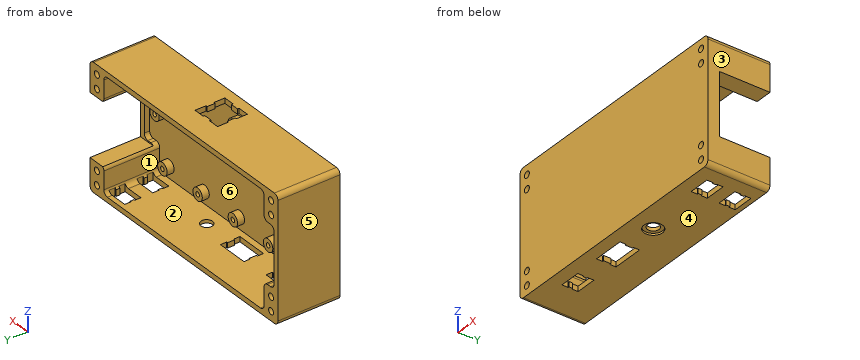
from build123d import *

# Parameters (mm, degrees)
EXTRUDE_1_DEPTH            = 40
CUT_EXTRUDE_1_DEPTH        = 36
EXTRUDE_2_DEPTH            = 36
SKETCH_4_R                 = 2.1
CUT_EXTRUDE_2_DEPTH        = 98.979589711
SKETCH_5_R                 = 4
SKETCH_5_R_2               = 1.5
EXTRUDE_3_DEPTH            = 4.5
PATTERN_LINEAR_1_COUNT     = 3
PATTERN_LINEAR_1_PITCH     = 30
PATTERN_LINEAR_1_COL_COUNT = 3
PATTERN_LINEAR_1_COL_PITCH = 30
SKETCH_6_R                 = 4
SKETCH_6_R_2               = 1.5
EXTRUDE_4_DEPTH            = 4.5
FILLET_1_R                 = 3
SKETCH_7_W                 = 40
SKETCH_7_H                 = 40
CUT_EXTRUDE_3_DEPTH        = 25
CUT_EXTRUDE_4_DEPTH        = 10
SKETCH_9_R                 = 3.75
CUT_EXTRUDE_5_DEPTH        = 3.3
SKETCH_10_R                = 6
CUT_EXTRUDE_6_DEPTH        = 1.2
CUT_EXTRUDE_7_REACH        = 122


with BuildPart() as part:
    # Эскиз1 → Бобышка-Вытянуть1 (new body)
    with BuildSketch(Plane(origin=(0, 0, 0), x_dir=(1, 0, 0), z_dir=(0, 1, 0))):
        with BuildLine():
            Line((-77, -40), (77, -40))
            ThreePointArc((77, -40), (79.121320344, -39.121320344), (80, -37))
            Line((80, -37), (80, 37))
            ThreePointArc((80, 37), (79.121320344, 39.121320344), (77, 40))
            Line((77, 40), (-77, 40))
            ThreePointArc((-77, 40), (-79.121320344, 39.121320344), (-80, 37))
            Line((-80, 37), (-80, -37))
            ThreePointArc((-80, -37), (-79.121320344, -39.121320344), (-77, -40))
        make_face()
    extrude(amount=EXTRUDE_1_DEPTH)

    # Эскиз2 → Вырез-Вытянуть1 (cut)
    with BuildSketch(Plane(origin=(0, 40, 0), x_dir=(1, 0, 0), z_dir=(0, 1, 0))):
        with BuildLine():
            Line((-75.75, -36.7), (75.75, -36.7))
            ThreePointArc((75.75, -36.7), (76.457106781, -36.407106781), (76.75, -35.7))
            Line((76.75, -35.7), (76.75, 35.7))
            ThreePointArc((76.75, 35.7), (76.457106781, 36.407106781), (75.75, 36.7))
            Line((75.75, 36.7), (-75.75, 36.7))
            ThreePointArc((-75.75, 36.7), (-76.457106781, 36.407106781), (-76.75, 35.7))
            Line((-76.75, 35.7), (-76.75, -35.7))
            ThreePointArc((-76.75, -35.7), (-76.457106781, -36.407106781), (-75.75, -36.7))
        make_face()
    extrude(amount=-CUT_EXTRUDE_1_DEPTH, mode=Mode.SUBTRACT)

    # Эскиз3 → Бобышка-Вытянуть2 (add)
    with BuildSketch(Plane(origin=(0, 4, 0), x_dir=(1, 0, 0), z_dir=(0, 1, 0))):
        with BuildLine():
            Line((-76.75, -36.7), (-68.2, -36.7))
            Line((-68.2, -36.7), (-68.2, -22.15))
            ThreePointArc((-68.2, -22.15), (-69.078679656, -20.028679656), (-71.2, -19.15))
            Line((-71.2, -19.15), (-76.75, -19.15))
            Line((-76.75, -19.15), (-76.75, -36.7))
        make_face()
        with BuildLine():
            Line((-68.2, 36.7), (-68.2, 22.15))
            ThreePointArc((-68.2, 22.15), (-69.078679656, 20.028679656), (-71.2, 19.15))
            Line((-71.2, 19.15), (-76.75, 19.15))
            Line((-76.75, 19.15), (-76.75, 36.7))
            Line((-76.75, 36.7), (-68.2, 36.7))
        make_face()
        with BuildLine():
            Line((76.75, 36.7), (68.2, 36.7))
            Line((68.2, 36.7), (68.2, 22.15))
            ThreePointArc((68.2, 22.15), (69.078679656, 20.028679656), (71.2, 19.15))
            Line((71.2, 19.15), (76.75, 19.15))
            Line((76.75, 19.15), (76.75, 36.7))
        make_face()
        with BuildLine():
            Line((68.2, -36.7), (68.2, -22.15))
            ThreePointArc((68.2, -22.15), (69.078679656, -20.028679656), (71.2, -19.15))
            Line((71.2, -19.15), (76.75, -19.15))
            Line((76.75, -19.15), (76.75, -36.7))
            Line((76.75, -36.7), (68.2, -36.7))
        make_face()
    extrude(amount=EXTRUDE_2_DEPTH)

    # Эскиз4 → Вырез-Вытянуть2 (cut, through all)
    with BuildSketch(Plane(origin=(0, 40, 0), x_dir=(1, 0, 0), z_dir=(0, 1, 0))):
        with Locations(Location((-74.15, -34, 0), (0, 0, 270))):
            Circle(SKETCH_4_R)
        with Locations(Location((-74.15, 34, 0), (0, 0, 90))):
            Circle(SKETCH_4_R)
        with Locations(Location((74.15, 34, 0), (0, 0, 270))):
            Circle(SKETCH_4_R)
        with Locations(Location((74.15, -34, 0), (0, 0, 90))):
            Circle(SKETCH_4_R)
        with Locations(Location((-74.15, -25.1, 0), (0, 0, 270))):
            Circle(SKETCH_4_R)
        with Locations(Location((-74.15, 25.1, 0), (0, 0, 90))):
            Circle(SKETCH_4_R)
        with Locations(Location((74.15, 25.1, 0), (0, 0, 270))):
            Circle(SKETCH_4_R)
        with Locations(Location((74.15, -25.1, 0), (0, 0, 90))):
            Circle(SKETCH_4_R)
    extrude(amount=-CUT_EXTRUDE_2_DEPTH, mode=Mode.SUBTRACT)

    # Эскиз5 → Бобышка-Вытянуть3 (add)
    # profile 1 of 2: a face of its own
    with BuildSketch(Plane(origin=(0, 4, 0), x_dir=(1, 0, 0), z_dir=(0, 1, 0))):
        with Locations(Location((0, -29, 0), (0, 0, 90))):
            Circle(SKETCH_5_R)
        with Locations(Location((0, -29, 0), (0, 0, 270))):
            Circle(SKETCH_5_R_2, mode=Mode.SUBTRACT)
    # profile 2 of 2: a face of its own
    with BuildSketch(Plane(origin=(0, 4, 0), x_dir=(1, 0, 0), z_dir=(0, 1, 0))):
        with Locations(Location((0, 29, 0), (0, 0, 90))):
            Circle(SKETCH_5_R)
        with Locations(Location((0, 29, 0), (0, 0, 270))):
            Circle(SKETCH_5_R_2, mode=Mode.SUBTRACT)
    extrude_3 = extrude(amount=EXTRUDE_3_DEPTH)

    # Линейный массив1: Бобышка-Вытянуть3 ×3
    with Locations(*[(i * PATTERN_LINEAR_1_PITCH, 0, 0) for i in range(1, PATTERN_LINEAR_1_COUNT)]):
        add(extrude_3)

    # Линейный массив1 col: Бобышка-Вытянуть3 ×3
    with Locations(*[(-i * PATTERN_LINEAR_1_COL_PITCH, 0, 0) for i in range(1, PATTERN_LINEAR_1_COL_COUNT)]):
        add(extrude_3)

    # Эскиз6 → Бобышка-Вытянуть4 (add)
    # profile 1 of 2: a face of its own
    with BuildSketch(Plane(origin=(0, 4, 0), x_dir=(1, 0, 0), z_dir=(0, 1, 0))):
        with Locations(Location((-68, 0, 0), (0, 0, 90))):
            Circle(SKETCH_6_R)
        with Locations(Location((-68, 0, 0), (0, 0, 270))):
            Circle(SKETCH_6_R_2, mode=Mode.SUBTRACT)
    # profile 2 of 2: a face of its own
    with BuildSketch(Plane(origin=(0, 4, 0), x_dir=(1, 0, 0), z_dir=(0, 1, 0))):
        with Locations(Location((68, 0, 0), (0, 0, 90))):
            Circle(SKETCH_6_R)
        with Locations(Location((68, 0, 0), (0, 0, 90))):
            Circle(SKETCH_6_R_2, mode=Mode.SUBTRACT)
    extrude(amount=EXTRUDE_4_DEPTH)

    # Скругление1
    fillet_1_edges = [part.edges().sort_by_distance(p)[0] for p in [
        (68.2, 22, 36.7),
        (76.75, 22, 19.15),
        (-76.75, 22, 19.15),
        (-68.2, 22, 36.7),
        (-68.2, 22, -36.7),
        (-76.75, 22, -19.15),
        (76.75, 22, -19.15),
        (68.2, 22, -36.7),
    ]]
    fillet(fillet_1_edges, radius=FILLET_1_R)

    # Эскиз7 → Вырез-Вытянуть3 (cut)
    with BuildSketch(Plane(origin=(80, 0, 0), x_dir=(0, 0, -1), z_dir=(1, 0, 0))):
        with Locations((0, 27.5)):
            Rectangle(SKETCH_7_W, SKETCH_7_H)
    extrude(amount=-CUT_EXTRUDE_3_DEPTH, mode=Mode.SUBTRACT)

    # Эскиз8 → Вырез-Вытянуть4 (cut)
    with BuildSketch(Plane(origin=(0, 0, -40), x_dir=(-1, 0, 0), z_dir=(0, 0, -1))):
        Polygon((-54.5, 18.9), (-67.9, 18.9), (-67.9, 14.9), (-67.2, 14.9), (-67.2, 12.5), (-67.9, 12.5), (-67.9, 8.5), (-54.5, 8.5), (-54.5, 12.5), (-55.2, 12.5), (-55.2, 14.9), (-54.5, 14.9), align=None)
        Polygon((55.5, 18.9), (42.1, 18.9), (42.1, 14.9), (42.8, 14.9), (42.8, 12.5), (42.1, 12.5), (42.1, 8.5), (55.5, 8.5), (55.5, 12.5), (54.8, 12.5), (54.8, 14.9), (55.5, 14.9), align=None)
        Polygon((-54.5, 36.9), (-67.9, 36.9), (-67.9, 32.9), (-67.2, 32.9), (-67.2, 30.5), (-67.9, 30.5), (-67.9, 26.5), (-54.5, 26.5), (-54.5, 30.5), (-55.2, 30.5), (-55.2, 32.9), (-54.5, 32.9), align=None)
    extrude(amount=-CUT_EXTRUDE_4_DEPTH, mode=Mode.SUBTRACT)

    # Эскиз9 → Вырез-Вытянуть5 (cut)
    with BuildSketch(Plane(origin=(0, 0, -40), x_dir=(-1, 0, 0), z_dir=(0, 0, -1))):
        with Locations((-14.7, 14.2)):
            Circle(SKETCH_9_R)
        Polygon((5.3, 20.5), (25.3, 20.5), (25.3, 16.5), (24.5, 16.5), (24.5, 11.9), (25.3, 11.9), (25.3, 7.9), (5.3, 7.9), (5.3, 11.9), (6.1, 11.9), (6.1, 16.5), (5.3, 16.5), align=None)
    extrude(amount=-CUT_EXTRUDE_5_DEPTH, mode=Mode.SUBTRACT)

    # Эскиз10 → Вырез-Вытянуть6 (cut)
    with BuildSketch(Plane(origin=(0, 0, -40), x_dir=(-1, 0, 0), z_dir=(0, 0, -1))):
        with Locations((-14.7, 14.2)):
            Circle(SKETCH_10_R)
    extrude(amount=-CUT_EXTRUDE_6_DEPTH, mode=Mode.SUBTRACT)

    # Эскиз11 → Вырез-Вытянуть7 (cut, up to next)
    with BuildSketch(Plane.XY.offset(40), mode=Mode.PRIVATE) as cut_extrude_7_sk1:
        Polygon((-9.6, 25.6), (-2.5, 25.6), (-2.5, 24.6), (2.5, 24.6), (2.5, 25.6), (9.6, 25.6), (9.6, 18.5), (8.6, 18.5), (8.6, 13.5), (9.6, 13.5), (9.6, 6.4), (2.5, 6.4), (2.5, 7.4), (-2.5, 7.4), (-2.5, 6.4), (-9.6, 6.4), (-9.6, 13.5), (-8.6, 13.5), (-8.6, 18.5), (-9.6, 18.5), align=None)
    cut_extrude_7_tool1 = extrude(cut_extrude_7_sk1.sketch, amount=-CUT_EXTRUDE_7_REACH, mode=Mode.PRIVATE) & part.part
    add(cut_extrude_7_tool1.solids().sort_by_distance((0, 16, 40))[0], mode=Mode.SUBTRACT)


solid = part.part
Can you work these out from the model? Positions are in its coordinate system, mm. Face numbers are marked on the shaded views. A direction names the side the tool comes from. Coordinates: 2 decimals unless noted, no trailing zeros. Write each loop counter-clockwise with the first axis right and the second up, starting at its lowest first coordinate (ties: lowest second). Pieces come first, ordered by that corner, then holes. Notation, with made-up numbers: (-27, -36) -> (-16, -36) arc R13 cw to (-16, -17) -> close; hole circle Ø11 at (-11, 81). An arc over 180 degrees is marked (long way). Write item = value, one per line.
(1) For pin 1 (3.5 mm diameter, centred on x = -30, z = 29, fed in from +Y); pin 2 (1.8 mm diameter, centred on x = 60, z = -29, fed in from +Y), each with a flat end and sliding along its axis, tell me the tip position at first contact or that it passes through.
Verdict:
pin_1 = 8.5
pin_2 = 4
(2) Imagine slicing it at C-C (x = -40.5). Please give me the cut outline in (y, z), and give its area (3 significant figures).
Verdict:
outline = (0, -40) -> (40, -40) -> (40, -36.7) -> (4, -36.7) -> (4, 36.7) -> (40, 36.7) -> (40, 40) -> (0, 40) -> close
area = 558 mm^2
(3) Imagine slicing it at B-B (z = 11). Please give me the cut outline in (x, y), and give its area (3 significant figures).
Verdict:
outline = (-80, 0) -> (80, 0) -> (80, 7.5) -> (76.75, 7.5) -> (76.75, 4) -> (-76.75, 4) -> (-76.75, 40) -> (-80, 40) -> close
area = 768 mm^2
(4) Thinking about a two-plate mould opening in Z: for the marked faces 1, 2, 3 and 4, which applies, +Z half, -Z half, draft (parallel to the pull), parting line (faces both ways), or undercut?
Verdict:
face_1 = undercut
face_2 = undercut
face_3 = draft
face_4 = -Z half
(5) Imagine slicing it at A-A (x = -18). Please give me the cut outline in (y, z).
Verdict:
outline = (0, -40) -> (7.9, -40) -> (7.9, -36.7) -> (4, -36.7) -> (4, 36.7) -> (40, 36.7) -> (40, 40) -> (0, 40) -> close; (20.5, -40) -> (40, -40) -> (40, -36.7) -> (20.5, -36.7) -> close
(6) Imagine slicing it at D-D (z = 0). Please give me the cut outline in (x, y).
Verdict:
outline = (-80, 0) -> (80, 0) -> (80, 7.5) -> (76.75, 7.5) -> (76.75, 4) -> (72, 4) -> (72, 7.5) -> (69.5, 7.5) -> (69.5, 4) -> (66.5, 4) -> (66.5, 7.5) -> (64, 7.5) -> (64, 4) -> (-64, 4) -> (-64, 8.5) -> (-66.5, 8.5) -> (-66.5, 4) -> (-69.5, 4) -> (-69.5, 8.5) -> (-72, 8.5) -> (-72, 4) -> (-76.75, 4) -> (-76.75, 40) -> (-80, 40) -> close
(7) If I drill on probe 1 along X at (y, z) = (7, 0); probe 2 along X at (y, z) = (20.5, 34); probe 3 along X at (y, z) = (26.5, -30), over which ranges is the centre line in solid material (lowest first)?
Verdict:
probe_1 = -80 to -76.75, -72 to -69.5, -66.5 to -64, 64 to 66.5, 69.5 to 72, 76.75 to 80
probe_2 = -80 to -76.25, -72.05 to -68.18, 68.18 to 72.05, 76.25 to 80
probe_3 = -80 to -68.2, 68.2 to 80
(8) On a 3-axis mill with a long thin cutter (end or side, diameter ignored), from which of +Z, -Z, +X, -X, +Y, -Y can I reach the whole of each face in a straight line? I mean the marked faces 5 and 6. Say none if no direction works.
Verdict:
face_5 = +Z, -Z, -X, +Y, -Y
face_6 = +Y
